Here's the drawing with two shaded views (mm, measured from the low corner). I have some questions. Give positions to 0.01 mm unless a question says otherwise; leave off trailing zeros. Order: outer loops, then holes, each group sorted by start corner. A loop starts at its lowest first (then second) coordinate and runs counter-clockwise, first axis right, second up. Notation, with made-up numbers: M -39.5,-25 L -5.5,-25 A22 cw -5.5,-9 Z; hole C 37,10.5 d6. An arc over 180 degrees is marked long. Use a Markdown table: item, result. Add a question column.
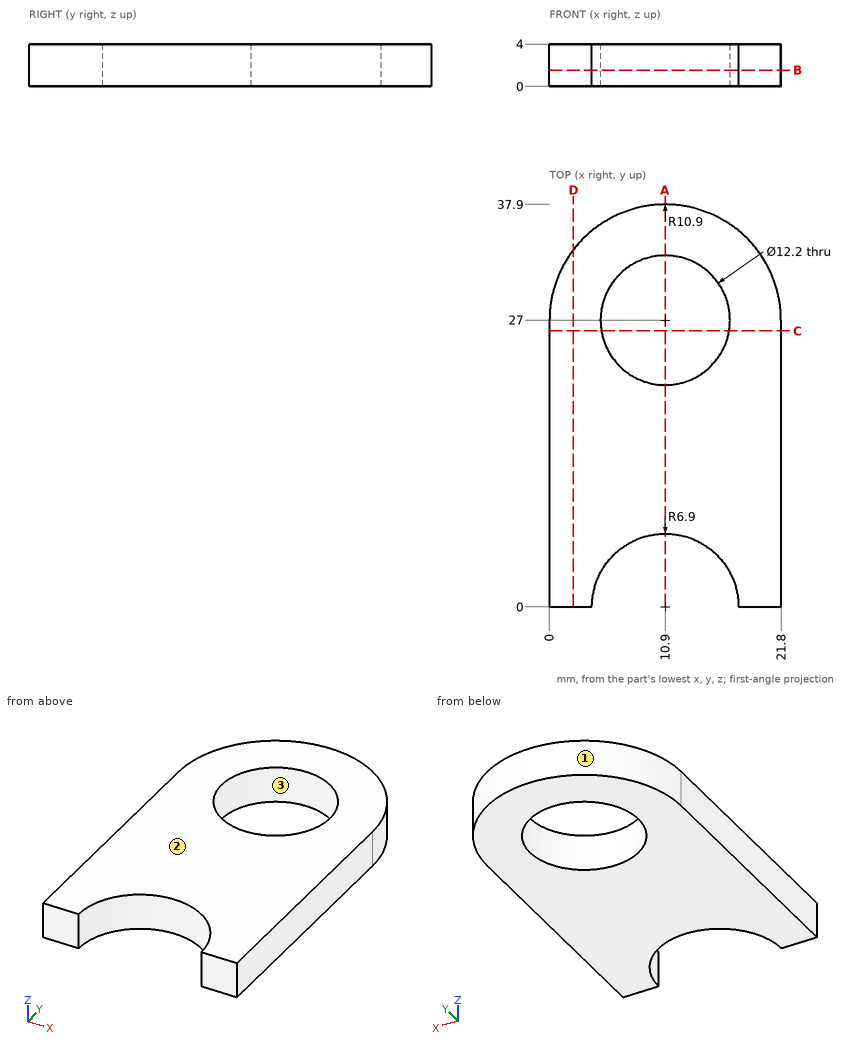
1) We'd pull the mould along Y, two halves only. Please class the marked faces 1, 2 and 3: pulls with the +Y half, pulls with the -Y half, needs draft (parallel to the pull), parting line crosses it, or undercut.
2) Suppose I cut it at D-D on x = 2.25. Please give me the cut outline in (y, z), and give its area (3 significant figures).
3) Please list where these lines run through material, in increasing order: line 1 (Y direction, x = 10.9, z = 1.6); line 2 (X direction, y = 26, z = 3.55); line 3 (Y direction, x = 6.5, z = 0.8). Write a range as from..to.
4) Suppose I cut it at C-C on y = 26. Please give me the cut outline in (x, z), and give its area (3 significant figures).
5) For pin 1 (2 mm diameter, centred on y = 31, z = 2.5, fed in from -X); pin 2 (10 mm diameter, centred on x = 10.9, y = 27, fed in from -Z), each with a flat end and sliding along its axis, tell me the tip position at first contact or that it passes through.
6) Suppose I cut it at A-A on x = 10.9. Please give me the cut outline in (y, z).
7) Suppose I cut it at B-B on z = 1.55. Please give me the cut outline in (x, y).
Values found:
| question | item | result |
|---|---|---|
| 1 | face 1 | pulls with the +Y half |
| 1 | face 2 | needs draft |
| 1 | face 3 | undercut |
| 2 | outline | M 0,0 L 33.63,0 L 33.63,4 L 0,4 Z |
| 2 | area | 135 mm^2 |
| 3 | line 1 | y = 6.9..20.9, 33.1..37.9 |
| 3 | line 2 | x = 0..4.88, 16.92..21.8 |
| 3 | line 3 | y = 5.32..22.78, 31.22..36.97 |
| 4 | outline | M 0,0 L 4.88,0 L 4.88,4 L 0,4 Z; M 16.92,0 L 21.8,0 L 21.8,4 L 16.92,4 Z |
| 4 | area | 39.1 mm^2 |
| 5 | pin 1 | stops at x = 0.42 |
| 5 | pin 2 | passes through |
| 6 | outline | M 6.9,0 L 20.9,0 L 20.9,4 L 6.9,4 Z; M 33.1,0 L 37.9,0 L 37.9,4 L 33.1,4 Z |
| 7 | outline | M 0,0 L 4,0 A6.9 cw 17.8,0 L 21.8,0 L 21.8,27 A10.9 ccw 0,27 Z; hole C 10.9,27 d12.2 |
